Can you work these out from the drawing? Everything is in mm from the part's minimum corner. A direction names the side the tool comes from. Round coordinates to 2 decimals unless told otherwise and drop trailing zeros. Loops run counter-clockwise (first coordinate to the right, second up) from the corner with the lowest first, then second, coordinate; pieces in that order, holes last. Notation, with made-up numbers: M 38,-10 L 79,-10 A23 cw 79,11 Z; hole C 73.25,-39 d2. An arc over 180 degrees is marked long. One line per question, with ' | ' between items. Start each with the question number.
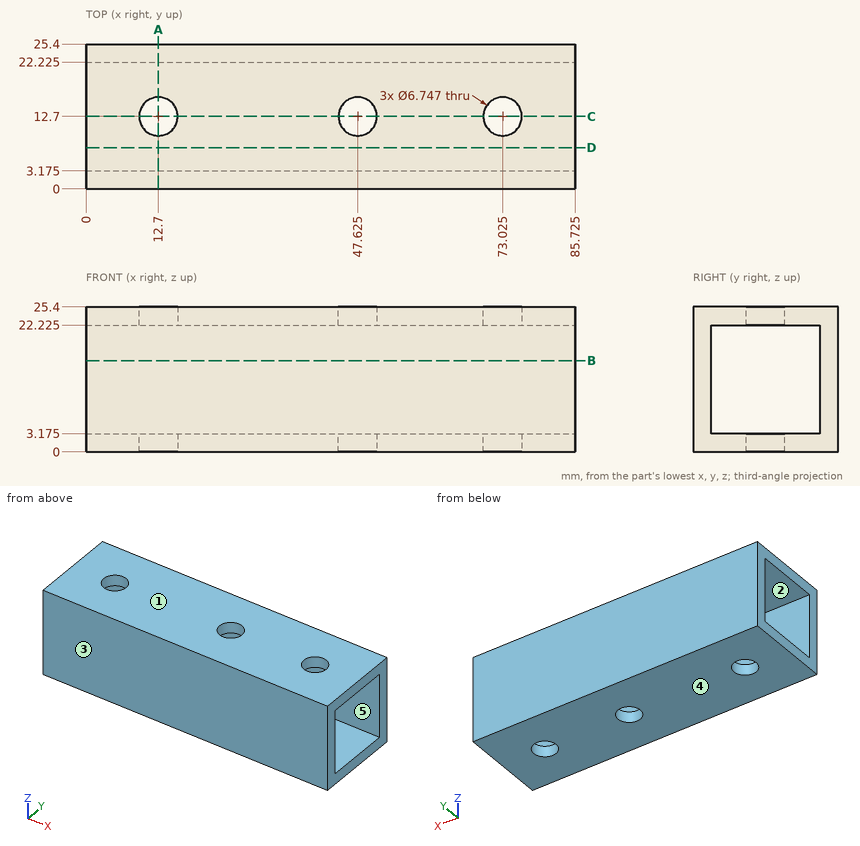
1) Imagine slicing it at B-B (z = 16). Write out the boundary of the cut face in (x, y) (3 decimals), then the cut area to 3 significant figures.
2) We'd pull the mould along Z, two halves only. Please class the marked faces 3, 4 and 5: pulls with the +Z half, pulls with the -Z half, needs draft (parallel to the pull), parting line crosses it, or undercut.
3) I'm going to push a flat-ended pin straight in: pin 1 Ø10 at (y, z) = (12, 11) entering from -X. Where does the tip first touch, or does it pass through?
4) Please list where these lines run through material, in increasing order: L1, parallel to Y at x = 77.5, z = 4.75 (3 decimals); L2, parallel to X at y = 11.5, z = 23.5 (1 decimal). Write a range as from..to.
5) Imagine slicing it at A-A (x = 12.7). Write out the boundary of the cut face in (y, z) (1 decimal).
6) Imagine slicing it at C-C (y = 12.7). State how many separate pieces and enclosed holes the cut face has, then the cut area to 3 significant figures.
7) For the marked faces 1 and 2, which set-ups out of +Z, -Z, +X, -X, +Y, -Y let a thin tool reach every point of the face, with its end or its side?
Results are:
1) outline: M 0,0 L 85.725,0 L 85.725,3.175 L 0,3.175 Z; M 0,22.225 L 85.725,22.225 L 85.725,25.4 L 0,25.4 Z | area: 544 mm²
2) face 3: needs draft | face 4: pulls with the -Z half | face 5: undercut
3) pin 1: through
4) L1: 0..3.175, 22.225..25.4 | L2: 0..9.5, 15.9..44.5, 50.8..69.9, 76.2..85.7
5) outline: M 0,0 L 9.3,0 L 9.3,3.2 L 3.2,3.2 L 3.2,22.2 L 9.3,22.2 L 9.3,25.4 L 0,25.4 Z; M 16.1,0 L 25.4,0 L 25.4,25.4 L 16.1,25.4 L 16.1,22.2 L 22.2,22.2 L 22.2,3.2 L 16.1,3.2 Z
6) separate pieces: 8 | enclosed holes: 0 | area: 416 mm²
7) face 1: +Z, +X, -X, +Y, -Y | face 2: +X, -X
